```python
from build123d import *

# Parameters (mm, degrees)
F2_R     = 4
F3_DEPTH = 70


with BuildPart() as f1:
    # F0 (on Right) → F1 (revolve)
    with BuildSketch(Plane.YZ):
        with BuildLine():
            Line((-10, 0), (0, 0))
            Line((0, 0), (0, 63.5))
            ThreePointArc((0, 63.5), (-3.409545, 63.879649), (-6.652067, 65))
            Line((-6.652067, 65), (-15, 65))
            Line((-15, 65), (-15, 16.8))
            Line((-15, 16.8), (-17.5, 16.8))
            Line((-17.5, 16.8), (-17.5, 10.8))
            Line((-17.5, 10.8), (-13, 10.8))
            Line((-13, 10.8), (-13, 9))
            Line((-13, 9), (-15, 9))
            Line((-15, 9), (-15, 1))
            Line((-15, 1), (-10, 1))
            Line((-10, 1), (-10, 0))
        make_face()
    revolve(axis=Axis((0, 0, 22.3796), (0, 0, -1)))

    # F2 (on Top) → F3 (cut)
    with BuildSketch(Plane.XY):
        Circle(F2_R)
    extrude(amount=F3_DEPTH, mode=Mode.SUBTRACT)


solid = f1.part
```
Part model, mm, in its own coordinate system. A direction names the side the tool comes from. Round coordinates to 2 decimals unless told otherwise and drop trailing zeros. Loops run counter-clockwise (first coordinate to the right, second up) from the corner with the lowest first, then second, coordinate; pieces in that order, holes last.
Item 1: Cut at B-B, the plane y = 11. Give the cut face in (x, z).
Item 2: Mould opens along Z. For faces 6 (the face through (-0.867, -3.905, 31.564)), 7 (the face through (-13, 3, 10.8)), 8 (the face through (-0.1, -4.3, 0)) say: +Z half, -Z half, draft (parallel to the pull), parting line (faces both ways), or undercut.
Item 3: 3-axis set-ups, long thin cutter, end or side, ignore diameter. For faces 1 (the face through (10, -3, 1)), 2 (the face through (-8, 13, 16.8)), 3 (the face through (7.91, 10.316, 9.887)), 4 (the face through (10.648, 13.887, 13.758)), 5 (the face through (6.5, 3.1, 65)): which of +Z, -Z, +X, -X, +Y, -Y reach the whole face in a straight line?
Item 4: Drop flat-ended pins along their axis: P1, Ø12, axis at y = 2, z = 53, coming from the -X side; P2, Ø7, axis at x = 0, y = 0, coming from the +Z side; P3, Ø10, axis at x = -10.5, y = 13.5, coming from the -Z side; P4, Ø10, axis at y = -8.5, z = 32, coming from the +X side. Give the stop position or say it passes through.
Item 5: Drill centre lines: line 1 (Y direction, x = 0, z = 31); line 2 (X direction, y = 0, z = 15); line 3 (Z direction, x = 9, y = 6.5). Where is each one in solid material? Low to high.
Item 6: Cut at A-A, the plane z = 21.5. Give the cut face in (x, y).
A:
1. outline: (-13.61, 10.8) - (-6.93, 10.8) - (-6.93, 9) - (-10.2, 9) - (-10.2, 1) - (10.2, 1) - (10.2, 9) - (6.93, 9) - (6.93, 10.8) - (13.61, 10.8) - (13.61, 16.8) - (10.2, 16.8) - (10.2, 65) - (-10.2, 65) - (-10.2, 16.8) - (-13.61, 16.8) - close
2. face 6: draft
2. face 7: undercut
2. face 8: -Z half
3. face 1: -Z
3. face 2: +Z
3. face 3: none
3. face 4: +Z, -Z
3. face 5: +Z, +X, -X, +Y, -Y
4. P1: stops at x = -15
4. P2: passes through
4. P3: stops at z = 1
4. P4: stops at x = 14.59
5. line 1: y = -15 to -4, 4 to 15
5. line 2: x = -17.5 to -4, 4 to 17.5
5. line 3: z = 1 to 65
6. outline: circle Ø30 at (0, 0); hole circle Ø8 at (0, 0)
